Can you work these out from the model? Positions are in its coordinate system, mm. Give positions to 0.01 mm unless a question says otherwise; leave off trailing zeros. Order: outer loops, then holes, each group sorted by start corner. A loop starts at its lowest first (then second) coordinate and runs counter-clockwise, first axis right, second up. Notation, with made-up numbers: (-33.75, 74) -> (-7.75, 74) arc R22 ccw to (-7.75, 111) -> close; hole circle Ø9 at (44.25, 0). An arc over 180 degrees is marked (long way). Answer as a JSON object with one key per item and string values.
```python
from build123d import *

# Parameters (mm, degrees)
F0_W     = 40
F0_H     = 40
F1_DEPTH = 280
F2_W     = 25
F2_H     = 30
F3_DEPTH = 20
F4_R     = 5


with BuildPart() as f1:
    # F0 (on Front) → F1 (new body)
    with BuildSketch(Plane.XZ):
        with Locations((-1e-06, -0.828695)):
            Rectangle(F0_W, F0_H)
    extrude(amount=F1_DEPTH)

    # F2 (on Top) → F3 (join)
    with BuildSketch(Plane.XY):
        with Locations((-1e-06, -35)):
            Rectangle(F2_W, F2_H)
        with Locations((-0.669636, -184.998505)):
            Rectangle(F2_W, F2_H)
    extrude(amount=F3_DEPTH)

    # F4
    f4_edges = [f1.edges().sort_by_distance(p)[0] for p in [
        (-1e-06, 0, 19.171305),
        (-20.000001, 0, -0.828695),
        (-1e-06, 0, -20.828695),
        (19.999999, 0, -0.828695),
        (19.999999, -140, -20.828695),
        (19.999999, -140, 19.171305),
        (19.999999, -280, -0.828695),
        (-20.000001, -140, -20.828695),
        (-1e-06, -280, -20.828695),
        (-20.000001, -140, 19.171305),
        (-20.000001, -280, -0.828695),
        (-1e-06, -280, 19.171305),
    ]]
    fillet(f4_edges, radius=F4_R)


solid = f1.part
```
1. If we section it at B-B on x = -1: Please give me the cut outline in (y, z).
Worked answers:
{"outline": "(-280, -15.83) arc R5 ccw to (-275, -20.83) -> (-5, -20.83) arc R5 ccw to (0, -15.83) -> (0, 14.17) arc R5 ccw to (-5, 19.17) -> (-20, 19.17) -> (-20, 20) -> (-50, 20) -> (-50, 19.17) -> (-170, 19.17) -> (-170, 20) -> (-200, 20) -> (-200, 19.17) -> (-275, 19.17) arc R5 ccw to (-280, 14.17) -> close"}
2. Please list where these lines run through material, in increasing order: L1, parallel to Z at x = 1, y = -126; L2, parallel to X at y = -94, z = 14.5; L3, parallel to X at y = -133, z = 16.5.
Worked answers:
{"L1": "-20.83 to 19.17", "L2": "-19.99 to 19.99", "L3": "-19.42 to 19.42"}
3. If we mould it in two halves opening along Y, with no side actions, what happens to faces 1 (the face through (0, -138, 19.171)), 2 (the face through (0.2, -1.4, -19.3)), 3 (the face through (-1, -185, 20))? For each: +Y half, -Y half, draft (parallel to the pull), parting line (faces both ways), or undercut.
Worked answers:
{"face 1": "undercut", "face 2": "+Y half", "face 3": "draft"}
4. Will this pin go through, and if not, where does the flat tip stop? pin 1 Ø4 at (x, y) = (6.5, -151.5) entering from +Z.
Worked answers:
{"pin 1": "z = 19.17"}
5. If we section it at A-A on y = -58.5: Please give me the cut outline in (x, z), then the cut area to 3 significant figures.
Worked answers:
{"outline": "(-20, -15.83) arc R5 ccw to (-15, -20.83) -> (15, -20.83) arc R5 ccw to (20, -15.83) -> (20, 14.17) arc R5 ccw to (15, 19.17) -> (-15, 19.17) arc R5 ccw to (-20, 14.17) -> close", "area": "1,580 mm²"}
